The model under review builds one solid part; all positions refer to its coordinate system, in mm. A direction names the side the tool comes from. Round coordinates to 2 decimals unless told otherwise and drop trailing zeros. Loops run counter-clockwise (first coordinate to the right, second up) from the corner with the lowest first, then second, coordinate; pieces in that order, holes last. Notation, with made-up numbers: M 22,53.5 L 56,53.5 A23 cw 56,81.5 Z; hole C 65.25,-36.5 d11. An arc over 180 degrees is marked long. One line per question, with ' | ' between items.
Autodesk Inventor part; units mm, degrees
ref_plane "YZ Plane" through (0, 0, 0) normal (1, 0, 0) x (0, 1, 0)
ref_plane "XZ Plane" through (0, 0, 0) normal (0, 1, 0) x (-1, 0, 0)
ref_plane "XY Plane" through (0, 0, 0) normal (0, 0, 1) x (1, 0, 0)
sketch "Sketch1" plane through (0, 0, 0) normal (0, 1, 0) x (-1, 0, 0)
  circle A0 centre (0, 0) radius 2
  dimension "d0" = 4
extrude "Extrusion1" add sketch "Sketch1" along normal blind 14
sketch "Sketch2" plane through (0, 14, 0) normal (0, 1, 0) x (1, 0, 0)
  circle A0 centre (0, 0) radius 2
  circle A1 centre (0, 0) radius 3.5
  dimension "d3" = 7
extrude "Extrusion2" add sketch "Sketch2" along normal blind 4 contours A0 | A1
sketch "Sketch3" plane through (0, 18, 0) normal (0, 1, 0) x (1, 0, 0)
  circle A0 centre (0, 0) radius 3.5
  line L0 (0, 1.8475) -> (1.6, 0.9238)
  line L1 (1.6, 0.9238) -> (1.6, -0.9238)
  line L2 (1.6, -0.9238) -> (0, -1.8475)
  line L3 (0, -1.8475) -> (-1.6, -0.9238)
  line L4 (-1.6, -0.9238) -> (-1.6, 0.9238)
  line L5 (-1.6, 0.9238) -> (0, 1.8475)
  dimension "d6" = 1.6
extrude "Extrusion3" cut sketch "Sketch3" against normal blind 3 contours L0 L1 L2 L3 L4 L5
thread "Thread1"
chamfer "Chamfer1" distance 0.25 angle 45 1 edges at (2, 0, 0)
properties part number "SHCS4x14"
1) Add section B-B on y = 11.75. State the section outline as (x, z) points.
Output values:
outline: C 0,0 d4
2) Mouldability with a two-part tool opening along X and no side actions: class faces 1 (the flat face through (1.6, 17, 0)), 2 (the flat face through (0, 0, 0)), 3 (the cylindrical face through (0, 7, 2)) as +X half, -X half, draft (parallel to the pull), parting line (faces both ways), or undercut.
Output values:
face 1: undercut | face 2: draft | face 3: parting line
3) Machinability: for faces 4 (the flat face through (-2, 18, 0)), 5 (the flat face through (0.79, 16.52, -1.39)), 6 (the flat face through (2, 14, 2)), which of the approach directions +Z, -Z, +X, -X, +Y, -Y give a long, thin tool a straight path to every point of the face, cutting with its end or side? Answer none if there is none.
Output values:
face 4: +Z, -Z, +X, -X, +Y | face 5: +Y | face 6: -Y
4) Insertion check: P1, Ø2, axis at y = 4, z = 1.5, coming from the -X side; P2, Ø4, axis at y = 4, z = 1.5, coming from the -X side. Each pin has a flat end and moves straight along its axis. Give the tip position at first contact, or say it passes through.
Output values:
P1: stops at x = -1.94 | P2: stops at x = -2
5) Add section D-D on z = 2.5. State the section outline as (x, y) points.
Output values:
outline: M -2.45,14 L 2.45,14 L 2.45,18 L -2.45,18 Z
6) Add section A-A on z = 0. State the section outline as (x, y) points.
Output values:
outline: M -3.5,14 L -2,14 L -2,0.25 L -1.75,0 L 1.75,0 L 2,0.25 L 2,14 L 3.5,14 L 3.5,18 L 1.6,18 L 1.6,15 L -1.6,15 L -1.6,18 L -3.5,18 Z
7) For line 1 (Y direction, x = -0.25, z = -3); line 2 (Y direction, x = 1, z = 0.25); line 3 (Z direction, x = -1, y = 3), list the stretches that pass through material, from the lowest coordinate up.
Output values:
line 1: y = 14 to 18 | line 2: y = 0 to 15 | line 3: z = -1.73 to 1.73
8) Add section C-C on x = 2.75. State the section outline as (y, z) points, then the cut area to 3 significant figures.
Output values:
outline: M 14,-2.17 L 18,-2.17 L 18,2.17 L 14,2.17 Z | area: 17.3 mm²
